from build123d import *

# Parameters (mm, degrees)
SKETCH4_R          = 3.81
SKETCH4_R_2        = 3.175
CUT_EXTRUDE1_DEPTH = 0.508
CUT_EXTRUDE2_START = -0.508
SKETCH5_R          = 3.81
SKETCH5_R_2        = 3.175
CUT_EXTRUDE2_DEPTH = 0.508
SKETCH7_R          = 6.35
SKETCH7_R_2        = 3.81
CUT_EXTRUDE3_DEPTH = 0.40005
CUT_EXTRUDE4_START = -0.40005
SKETCH8_R          = 6.35
SKETCH8_R_2        = 3.81
CUT_EXTRUDE4_DEPTH = 0.40005


with BuildPart() as part:
    # Sketch1 → Revolve1 (revolve)
    with BuildSketch(Plane.XY, mode=Mode.PRIVATE) as revolve1_sk:
        with BuildLine():
            Line((0, 1.5875), (4.8133, 1.5875))
            Line((4.8133, 1.5875), (4.8133, 6.35))
            Line((4.8133, 6.35), (2.860814617, 4.987821073))
            ThreePointArc((2.860814617, 4.987821073), (2.40665, 4.84505), (1.952485383, 4.987821073))
            Line((1.952485383, 4.987821073), (0, 6.35))
            Line((0, 6.35), (0, 1.5875))
        make_face()
    revolve(revolve1_sk.sketch.rotate(Axis((0, 0, 0), (1, 0, 0)), 90), axis=Axis((0, 0, 0), (1, 0, 0)))

    # Sketch4 → Cut-Extrude1 (cut)
    with BuildSketch(Plane(origin=(4.8133, 0, 0), x_dir=(0, 0, -1), z_dir=(1, 0, 0))):
        Circle(SKETCH4_R)
        Circle(SKETCH4_R_2, mode=Mode.SUBTRACT)
    extrude(amount=-CUT_EXTRUDE1_DEPTH, mode=Mode.SUBTRACT)

    # Sketch5 → Cut-Extrude2 (cut)
    with BuildSketch(Plane.ZY.offset(CUT_EXTRUDE2_START)):
        with Locations(Location((0, 0, 0), (0, 0, 180))):
            Circle(SKETCH5_R)
        with Locations(Location((0, 0, 0), (0, 0, 180))):
            Circle(SKETCH5_R_2, mode=Mode.SUBTRACT)
    extrude(amount=CUT_EXTRUDE2_DEPTH, mode=Mode.SUBTRACT)

    # Sketch7 → Cut-Extrude3 (cut)
    with BuildSketch(Plane(origin=(4.8133, 0, 0), x_dir=(0, 0, -1), z_dir=(1, 0, 0))):
        Circle(SKETCH7_R)
        Circle(SKETCH7_R_2, mode=Mode.SUBTRACT)
    extrude(amount=-CUT_EXTRUDE3_DEPTH, mode=Mode.SUBTRACT)

    # Sketch8 → Cut-Extrude4 (cut)
    with BuildSketch(Plane.ZY.offset(CUT_EXTRUDE4_START)):
        Circle(SKETCH8_R)
        Circle(SKETCH8_R_2, mode=Mode.SUBTRACT)
    extrude(amount=CUT_EXTRUDE4_DEPTH, mode=Mode.SUBTRACT)


solid = part.part
Could you check a few things on this model? Use its own coordinates, in mm. A direction names the side the tool comes from. Round coordinates to 2 decimals unless told otherwise and drop trailing zeros. Order: outer loops, then holes, each group sorted by start corner. A loop starts at its lowest first (then second) coordinate and runs counter-clockwise, first axis right, second up.
Q1. Which directions (+Z, -Z, +X, -X, +Y, -Y) give clear straight access to the entire face, cutting with the end or side of a thin tool? Please do faces 1 (the face through (4.813, 1.4, -1.4)), 2 (the face through (4.413, 3, -3)), 3 (the face through (0.3, 2.8, -1.5)).
Geometry says:
face 1: +Z, -Z, +X, +Y, -Y
face 2: +X
face 3: -X
Q2. Please list where these lines run through material, in increasing order: probe 1 along Y at (x, z) = (1.75, 0.5); probe 2 along X at (y, z) = (0.25, 5.25); probe 3 along X at (y, z) = (4.5, 0.75).
Geometry says:
probe 1: y = -5.1 to -1.51, 1.51 to 5.1
probe 2: x = 0.4 to 1.57, 3.25 to 4.41
probe 3: x = 0.4 to 4.41
Q3. I'm going to push flat-ended pins straight in: P1, Ø1.5, axis at x = 1.5, z = -3.5, coming from the +Y side; P2, Ø1.5, axis at x = 1.5, z = 4, coming from the +Y side; P3, Ø2, axis at x = 1, y = -2.5, coming from the -Z side. Where does each tip first touch, or does it pass through?
Geometry says:
P1: stops at y = 4.84
P2: stops at y = 4.49
P3: stops at z = -5.83
Q4. Imagine slicing it at D-D, the plane x = 3.1. List the corners of the cut face in (y, z) for me (1 decimal).
Geometry says:
outline: circle Ø10.3 at (0, 0); hole circle Ø3.2 at (0, 0)
Q5. Imagine slicing it at C-C, the plane x = 3.8. List the corners of the cut face in (y, z) for me (1 decimal), then the cut area to 3 significant figures.
Geometry says:
outline: circle Ø11.3 at (0, 0); hole circle Ø3.2 at (0, 0)
area: 92.1 mm2
Q6. Thinking about a two-plate mould opening in Y: for faces 4 (the face through (4.56, -3.1, 0.69)), 5 (the face through (0.4, 3, 3)), which applies, released by +Y, released by -Y, zero draft, split by the parting line, or undercut?
Geometry says:
face 4: undercut
face 5: zero draft
